```python
from build123d import *

# Parameters (mm, degrees)
SKETCH1_W           = 120
SKETCH1_H           = 250
BOSS_EXTRUDE1_DEPTH = 100
CUT_EXTRUDE2_DEPTH  = 171.953209973
SKETCH3_R           = 25
CUT_EXTRUDE5_DEPTH  = 201.062490237
CUT_EXTRUDE8_DEPTH  = 60
SKETCH6_R           = 25
BOSS_EXTRUDE2_DEPTH = 120.5
FILLET1_R           = 12


with BuildPart() as part:
    # Sketch1 → Boss-Extrude1 (new body)
    with BuildSketch(Plane(origin=(0, 0, 0), x_dir=(1, 0, 0), z_dir=(0, 1, 0))):
        Rectangle(SKETCH1_W, SKETCH1_H)
    extrude(amount=BOSS_EXTRUDE1_DEPTH)

    # Sketch2 → Cut-Extrude2 (cut, through all)
    with BuildSketch(Plane(origin=(0, 100, 0), x_dir=(1, 0, 0), z_dir=(0, 1, 0))):
        with BuildLine():
            Line((-30, 50.498344353), (-30, 124.968053811))
            Line((-30, 124.968053811), (30, 124.968053811))
            Line((30, 124.968053811), (30, 50.498344353))
            ThreePointArc((30, 50.498344353), (33.533981136, 32.034620706), (43.636363636, 16.180915101))
            ThreePointArc((43.636363636, 16.180915101), (55.759222691, -2.84353176), (60, -25.000000292))
            Line((60, -25.000000292), (60, 125))
            Line((60, 125), (-60, 125))
            Line((-60, 125), (-60, -25))
            ThreePointArc((-60, -25), (-55.759222637, -2.843531624), (-43.636363636, 16.180915101))
            ThreePointArc((-43.636363636, 16.180915101), (-33.533981136, 32.034620706), (-30, 50.498344353))
        make_face()
        with BuildLine():
            ThreePointArc((30, -21), (21.213203436, 0.213203436), (0, 9))
            ThreePointArc((0, 9), (-21.213203436, 0.213203436), (-30, -21))
            Line((-30, -21), (-30, -125))
            Line((-30, -125), (30, -125))
            Line((30, -125), (30, -21))
        make_face()
    extrude(amount=-CUT_EXTRUDE2_DEPTH, mode=Mode.SUBTRACT)

    # Sketch3 → Cut-Extrude5 (cut, through all)
    # profile 1 of 2: a face of its own
    with BuildSketch(Plane(origin=(60, 0, 0), x_dir=(0, 0, -1), z_dir=(1, 0, 0))):
        Polygon((124.968053811, 0), (124.968053811, 100), (50.498344353, 100), (16.180915101, 100), (-25, 100), (-125, 100), (-125, 0), (-25, 0), (16.180915101, 0), (50.498344353, 0), align=None)
        with BuildLine():
            Line((124.958839528, 80), (-24.009804864, 80))
            ThreePointArc((-24.009804864, 80), (-33.138514156, 81.726266594), (-41.006536576, 86.666666667))
            ThreePointArc((-41.006536576, 86.666666667), (-125, 50), (-41.006536576, 13.333333333))
            ThreePointArc((-41.006536576, 13.333333333), (-33.138514156, 18.273733406), (-24.009804864, 20))
            Line((-24.009804864, 20), (124.958839528, 20))
            Line((124.958839528, 20), (124.958839528, 80))
        make_face(mode=Mode.SUBTRACT)
    # profile 2 of 2: a face of its own
    with BuildSketch(Plane(origin=(60, 0, 0), x_dir=(0, 0, -1), z_dir=(1, 0, 0))):
        with Locations((-75, 50)):
            Circle(SKETCH3_R)
    extrude(amount=-CUT_EXTRUDE5_DEPTH, mode=Mode.SUBTRACT)

    # Sketch4 → Cut-Extrude8 (cut)
    with BuildSketch(Plane(origin=(0, 0, -124.958839528), x_dir=(-1, 0, 0), z_dir=(0, 0, -1))):
        Polygon((11.94, 80), (30, 61.94), (30, 80), align=None)
        Polygon((30, 38.06), (11.94, 20), (30, 20), align=None)
        Polygon((-11.94, 20), (-30, 38.06), (-30, 20), align=None)
        Polygon((-30, 61.94), (-11.94, 80), (-30, 80), align=None)
    extrude(amount=-CUT_EXTRUDE8_DEPTH, mode=Mode.SUBTRACT)

    # Sketch6 → Boss-Extrude2 (add)
    with BuildSketch(Plane(origin=(0, 0, -124.958839528), x_dir=(-1, 0, 0), z_dir=(0, 0, -1))):
        with Locations((0, 50)):
            Circle(SKETCH6_R)
    extrude(amount=BOSS_EXTRUDE2_DEPTH)

    # Fillet1
    fillet1_edges = [part.edges().sort_by_distance(p)[0] for p in [
        (-20.97, 70.97, -64.958839528),
        (-20.97, 29.03, -64.958839528),
        (20.97, 29.03, -64.958839528),
        (20.97, 70.97, -64.958839528),
    ]]
    fillet(fillet1_edges, radius=FILLET1_R)


solid = part.part
```
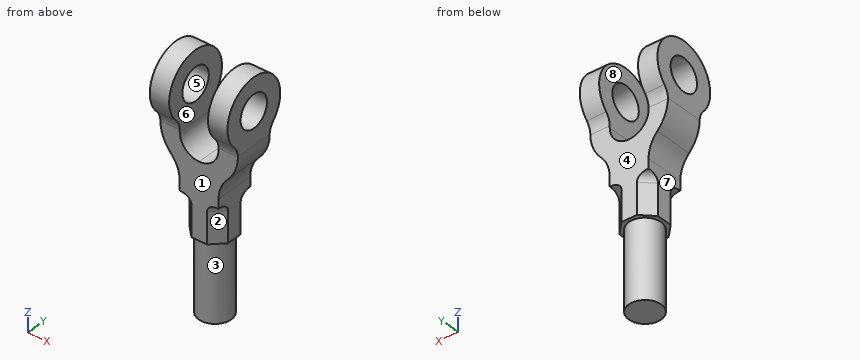
For this review, take the finished solid that the model builds, in its own axes (mm). Face numbers are marked on the shaded views. A direction names the side the tool comes from. Round coordinates to 2 decimals unless told otherwise and drop trailing zeros. Write each loop counter-clockwise with the first axis right and the second up, starting at its lowest first coordinate (ties: lowest second). Pieces come first, ordered by that corner, then holes. Notation, with made-up numbers: (-31, -8.75) -> (-4, -8.75) arc R23 cw to (-4, 12.25) -> close; hole circle Ø4 at (21.25, 60). An arc over 180 degrees is marked (long way). One line per question, with ' | ' between items. Start each with the question number.
(1) Insertion check: P1, Ø1.5, axis at y = 75.5, z = -91.5, coming from the +X side; P2, Ø1.2, axis at x = -29.5, y = 20.5, coming from the -Z side; P3, Ø4, axis at x = -37.5, y = 76, coming from the -Z side; P4, Ø4, axis at x = -26, y = 55, coming from the -Z side. Each pin has a flat end and moves straight along its axis. Give the tip position at first contact, or say it passes through.
(2) Add section B-B, the plane z = 75. Write out the cut boundary in (x, y).
(3) Tool access review of the marked faces 1, 2, 3 and 4: name each direction out of +Z, -Z, +X, -X, +Y, -Y from which nothing blocks a thin tool from reaching the whole face with its end or side.
(4) Add section A-A, the plane y = 50. Write out the cut boundary in (x, z), plus the area to 3 significant figures.
(5) For line 1 along Y through (x, z) = (-48, 75); line 2 along X through (y, z) = (23.5, 105); line 3 along Z through (x, y) = (-52.5, 58.5), list the stretches that pass through material, from the lowest coordinate up. Write a range as from..to.
(6) Add section D-D, the plane z = -222.5. Write out the cut boundary in (x, y), plus the area to 3 significant figures.
(7) Mouldability with a two-part tool opening along X and no side actions: class the marked faces 5, 6, 7 and 8 as released by +X, released by -X, zero draft, split by the parting line, or undercut.
(8) Add section C-C, the plane x = -48. Write out the cut boundary in (y, z), plus the area to 3 significant figures.
Answer list:
1) P1: x = 17.19 | P2: z = -64.97 | P3: z = -27.7 | P4: z = -245.46
2) outline: (-60, 0) -> (-30, 0) -> (-30, 25) -> (-60, 25) -> close; (-60, 75) -> (-30, 75) -> (-30, 100) -> (-60, 100) -> close; (30, 0) -> (60, 0) -> (60, 25) -> (30, 25) -> close; (30, 75) -> (60, 75) -> (60, 100) -> (30, 100) -> close
3) face 1: -Z, +X, -X, -Y | face 2: -Z, +X, -Y | face 3: -Z | face 4: -Z, +X, -X, +Y
4) outline: (-60, 25) arc R60 ccw to (-43.64, -16.18) arc R50 cw to (-30, -50.5) -> (-30, -124.96) -> (-25, -124.96) -> (-25, -245.46) -> (25, -245.46) -> (25, -124.96) -> (30, -124.96) -> (30, -50.5) arc R50 cw to (43.64, -16.18) arc R60 ccw to (60, 25) -> (60, 50) -> (30, 50) -> (30, 21) arc R30 cw to (-30, 21) -> (-30, 50) -> (-60, 50) -> close; (-60, 100) -> (-30, 100) -> (-30, 125) -> (-60, 125) -> close; (30, 100) -> (60, 100) -> (60, 125) -> (30, 125) -> close | area: 18,700 mm²
5) line 1: 0..25, 75..100 | line 2: -60..-30, 30..60 | line 3: -4.05..51.49, 98.51..124.27
6) outline: circle Ø50 at (0, 50) | area: 1,960 mm²
7) face 5: zero draft | face 6: undercut | face 7: released by -X | face 8: undercut
8) outline: (13.33, 41.01) arc R25 cw to (20, 24.01) -> (20, -11) -> (80, -11) -> (80, 24.01) arc R25 cw to (86.67, 41.01) arc R50 ccw (long way) to start; hole circle Ø50 at (50, 75) | area: 8,270 mm²
